CAD build for the part. Positions are in the model's coordinates, mm. A direction names the side the tool comes from. Coordinates: 2 decimals unless noted, no trailing zeros. Loops run counter-clockwise (first coordinate to the right, second up) from the corner with the lowest first, then second, coordinate; pieces in that order, holes last. Notation, with made-up numbers: (44.5, 4) - (70.5, 4) arc R15 ccw to (70.5, 12) - close; hole circle Ø9 at (38.25, -9.5). An arc over 180 degrees is marked (long way). Put each result on its own line as item: value.
```python
from build123d import *

# Parameters (mm, degrees)
SKETCH_1_W          = 130.5
SKETCH_1_H          = 130.5
EXTRUDE_1_DEPTH     = 330
SKETCH_8_R          = 56.25
CUT_EXTRUDE_2_DEPTH = 315


with BuildPart() as part:
    # 草图1 → 凸台-拉伸1 (new body)
    with BuildSketch(Plane(origin=(0, 0, 0), x_dir=(0, 0, -1), z_dir=(1, 0, 0))):
        Rectangle(SKETCH_1_W, SKETCH_1_H)
    extrude(amount=EXTRUDE_1_DEPTH)

    # 草图8 → 切除-拉伸2 (cut)
    with BuildSketch(Plane.ZY):
        Circle(SKETCH_8_R)
    extrude(amount=-CUT_EXTRUDE_2_DEPTH, mode=Mode.SUBTRACT)

    # 草图26 → 切除-旋转3 (revolve, cut)
    with BuildSketch(Plane(origin=(0, 0, 0), x_dir=(-1, 0, 0), z_dir=(0, 0, -1))):
        Polygon((-315, 0), (-315, 22.5), (-316, 22.5), (-327, 53.439293368), (-330, 53.439293368), (-330, 0), align=None)
    revolve(axis=Axis((315, 0, 0), (-1, 0, 0)), mode=Mode.SUBTRACT)


solid = part.part
```
Q1. Wall check: L1, parallel to Y at x = 211, z = 0; L2, parallel to Z at x = 315.3, y = 0; L3, parallel to Z at x = 328, y = 0. Give the ranges that are in metal, low to high. Write a range as from..to.
Determined:
L1: -65.25..-56.25, 56.25..65.25
L2: -65.25..-22.5, 22.5..65.25
L3: -65.25..-53.44, 53.44..65.25
Q2. Pin check, flat tip, straight feed: pin 1 Ø6 at (y, z) = (-42, 14.5) entering from -X. Stop position of the tip, or through.
Determined:
pin 1: x = 315
Q3. Mould opens along Z. For faces 4 (the flat face through (163, -1, -65.25)), 5 (the flat face through (163, -1, 65.25)), 6 (the flat face through (330, 1, 59)), 7 (the conical face through (316.688, -5.297, 23.854)) say: +Z half, -Z half, draft (parallel to the pull), parting line (faces both ways), or undercut.
Determined:
face 4: -Z half
face 5: +Z half
face 6: draft
face 7: undercut
Q4. Slice it at A-A, the plane y = 0. Give the cut face in (x, z), then the cut area to 3 significant figures.
Determined:
outline: (0, -65.25) - (330, -65.25) - (330, -53.44) - (327, -53.44) - (316, -22.5) - (315, -22.5) - (315, -56.25) - (0, -56.25) - close; (0, 56.25) - (315, 56.25) - (315, 22.5) - (316, 22.5) - (327, 53.44) - (330, 53.44) - (330, 65.25) - (0, 65.25) - close
area: 6,430 mm2
Q5. Tool access for faces 1 (the cylindrical face through (328.521, 50.972, -16.052)), 2 (the cylindrical face through (155.295, 2.473, -56.196)), 3 (the flat face through (0, 1, 59)): list every direction of +Z, -Z, +X, -X, +Y, -Y with a clear straight run to the whole face (end or side of a thin tool).
Determined:
face 1: +X
face 2: -X
face 3: +Z, -Z, -X, +Y, -Y
Q6. Slice it at C-C, the plane x = 20. Give the cut face in (y, z).
Determined:
outline: (-65.25, -65.25) - (65.25, -65.25) - (65.25, 65.25) - (-65.25, 65.25) - close; hole circle Ø112.5 at (0, 0)
